CAD build for the part. Positions are in the model's coordinates, mm. A direction names the side the tool comes from. Round coordinates to 2 decimals unless told otherwise and drop trailing zeros. Order: outer loops, then holes, each group sorted by start corner. A loop starts at its lowest first (then second) coordinate and runs counter-clockwise, first axis right, second up. Notation, with made-up numbers: (-9, 83.25) - (27, 83.25) arc R14 cw to (27, 92.25) - close; hole circle Ø1 at (-10.5, 87). An arc over 180 degrees is marked (long way). Write item = value, one per line.
from build123d import *

# Parameters (mm, degrees)
SKETCH_1_R                   = 52.5
EXTRUDE_1_DEPTH              = 20
CUT_EXTRUDE_START            = -12
SKETCH_3_R                   = 52.5
SKETCH_3_R_2                 = 18
CUT_EXTRUDE_1_DEPTH          = 12
SKETCH_5_R                   = 15.25
CUT_EXTRUDE_3_DEPTH          = 17.5
HOLE_WIZARD_M4_1_D           = 4.5
HOLE_WIZARD_M4_1_CBORE_D     = 8
HOLE_WIZARD_M4_1_CBORE_DEPTH = 4.6
PATTERN_CIRCULAR_1_COUNT     = 6
FILLET_2_R                   = 7
FILLET_3_R                   = 5


with BuildPart() as part:
    # 草图1 → 凸台-拉伸1 (new body)
    with BuildSketch(Plane.XY):
        Circle(SKETCH_1_R)
    extrude(amount=EXTRUDE_1_DEPTH)

    # 草图3 → 切除-拉伸1 (cut)
    with BuildSketch(Plane.XY.offset(20).offset(CUT_EXTRUDE_START)):
        Circle(SKETCH_3_R)
        Circle(SKETCH_3_R_2, mode=Mode.SUBTRACT)
    extrude(amount=CUT_EXTRUDE_1_DEPTH, mode=Mode.SUBTRACT)

    # 草图5 → 切除-拉伸3 (cut)
    with BuildSketch(Plane(origin=(0, 0, 0), x_dir=(-1, 0, 0), z_dir=(0, 0, -1))):
        with Locations((0, 0.647267044)):
            Circle(SKETCH_5_R)
    extrude(amount=-CUT_EXTRUDE_3_DEPTH, mode=Mode.SUBTRACT)

    # M4 六角圆柱头螺钉的柱形沉头孔1 (through all)
    with Locations(Plane.XY.offset(8)):
        with Locations((33.394511176, 27.088865302)):
            hole_wizard_m4_1 = CounterBoreHole(HOLE_WIZARD_M4_1_D / 2, HOLE_WIZARD_M4_1_CBORE_D / 2, HOLE_WIZARD_M4_1_CBORE_DEPTH)

    # 阵列(圆周)1: M4 六角圆柱头螺钉的柱形沉头孔1 ×6 about axis
    pattern_circular_1_axis = Axis((0, 0, 0), (0, 0, 1))
    for i in range(1, PATTERN_CIRCULAR_1_COUNT):
        add(hole_wizard_m4_1.rotate(pattern_circular_1_axis, i * 360 / PATTERN_CIRCULAR_1_COUNT), mode=Mode.SUBTRACT)

    # 圆角2
    fillet_2_edges = [part.edges().sort_by_distance(p)[0] for p in [
        (-18, 0, 20),
    ]]
    fillet(fillet_2_edges, radius=FILLET_2_R)

    # 圆角3
    fillet_3_edges = [part.edges().sort_by_distance(p)[0] for p in [
        (-52.5, 0, 8),
    ]]
    fillet(fillet_3_edges, radius=FILLET_3_R)


solid = part.part
(1) Probe line 1 along Z through (x, y) = (12, 26.5); line 2 along Z through (x, y) = (3, 10); line 3 along X through (y, z) = (-45.5, 5.5). List the from-to ranges inside material, lowest first.
Solved:
line_1 = 0 to 8
line_2 = 17.5 to 20
line_3 = -24.82 to 4.16, 9.37 to 24.82
(2) Drop flat-ended pins along their axis: pin 1 (13 mm diameter, centred on x = -33.39, y = -27.09, fed in from +Z); pin 2 (7 mm diameter, centred on x = 33.39, y = 27.09, fed in from +Z); pin 3 (2 mm diameter, centred on y = -2, z = 7.5, fed in from +X); pin 4 (4 mm diameter, centred on x = -40.16, y = 15.38, fed in from -Z). Give the stop position or say it passes through.
Solved:
pin_1 = 8
pin_2 = 3.4
pin_3 = 51.03
pin_4 = through
(3) Tool access for faces 1 (the flat face through (-4, 43, 3.4)), 2 (the cylindrical face through (12.102, -8.632, 8.628)), 3 (the cylindrical face through (-7.055, 40.234, 1.676)): list every direction of +Z, -Z, +X, -X, +Y, -Y with a clear straight run to the whole face (end or side of a thin tool).
Solved:
face_1 = +Z
face_2 = -Z
face_3 = +Z, -Z
(4) Band-saw the part on B-B on z = 14.5. List the corners of the cut face in (x, y), plus the area to 3 significant figures.
Solved:
outline = circle Ø35.67 at (0, 0); hole circle Ø30.5 at (0, 0.65)
area = 269 mm²
(5) Band-saw the part on A-A on x = 0. List the corners of the cut face in (y, z).
Solved:
outline = (-52.5, 0) - (-14.6, 0) - (-14.6, 17.5) - (15.9, 17.5) - (15.9, 0) - (52.5, 0) - (52.5, 3) arc R5 ccw to (47.5, 8) - (18, 8) - (18, 13) arc R7 ccw to (11, 20) - (-11, 20) arc R7 ccw to (-18, 13) - (-18, 8) - (-47.5, 8) arc R5 ccw to (-52.5, 3) - close
